Model file for the job. Use its own axes, mm. Face numbers are marked on the shaded views. A direction names the side the tool comes from. Round coordinates to 2 decimals unless told otherwise and drop trailing zeros. Order: outer loops, then holes, each group sorted by start corner. A loop starts at its lowest first (then second) coordinate and runs counter-clockwise, first axis right, second up. Notation, with made-up numbers: (79.5, 14) - (137.5, 14) arc R21 cw to (137.5, 50) - close; hole circle Ø7 at (18.5, 27). An arc over 180 degrees is marked (long way). Write item = value, one per line. Start each with the question number.
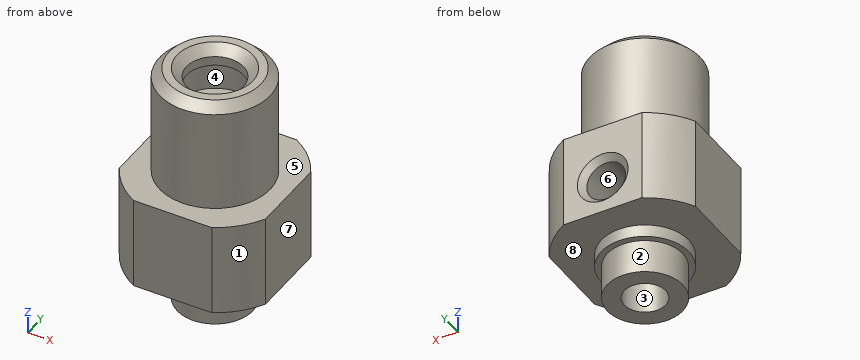
from build123d import *

# Parameters (mm, degrees)
CUT_EXTRUDE2_REACH              = 24
M5X0_8_TAPPED_HOLE1_D           = 4.2
M5X0_8_TAPPED_HOLE1_DEPTH       = 7
M5X0_8_TAPPED_HOLE1_CSINK_D     = 5.5
M5X0_8_TAPPED_HOLE1_CSINK_ANGLE = 90


with BuildPart() as part:
    # Sketch1 → Revolve1 (revolve)
    with BuildSketch(Plane(origin=(0, 0, 0), x_dir=(0, 0, -1), z_dir=(1, 0, 0))):
        Polygon((-12.5, 3.1), (-13.5, 4.1), (-13.5, 5), (-12.5, 6), (-1.5, 6), (-1.5, 9), (8.5, 9), (8.5, 4.75), (9.85, 4.75), (9.85, 4.1), (13.5, 4.1), (13.5, 2.25), (-8, 2.25), (-8, 4.15), (-11.5, 4.15), (-11.5, 3.1), align=None)
    revolve(axis=Axis((0, 0, 0), (0, 0, -1)))

    # Sketch2 → Cut-Extrude2 (cut, up to next)
    with BuildSketch(Plane(origin=(0, 0, -8.5), x_dir=(-1, 0, 0), z_dir=(0, 0, -1)), mode=Mode.PRIVATE) as cut_extrude2_sk1:
        with BuildLine():
            ThreePointArc((4.242180306, 7.9375), (0, 9), (-4.242180306, 7.9375))
            Line((-4.242180306, 7.9375), (4.242180306, 7.9375))
        make_face()
    cut_extrude2_tool1 = extrude(cut_extrude2_sk1.sketch, amount=-CUT_EXTRUDE2_REACH, mode=Mode.PRIVATE) & part.part
    add(cut_extrude2_tool1.solids().sort_by_distance((0, 8.364726, -8.5))[0], mode=Mode.SUBTRACT)
    # Sketch2 → Cut-Extrude2 (cut, up to next)
    with BuildSketch(Plane(origin=(0, 0, -8.5), x_dir=(-1, 0, 0), z_dir=(0, 0, -1)), mode=Mode.PRIVATE) as cut_extrude2_sk2:
        with BuildLine():
            Line((-7.9375, -4.242180306), (-7.9375, 4.242180306))
            ThreePointArc((-7.9375, 4.242180306), (-9, 0), (-7.9375, -4.242180306))
        make_face()
    cut_extrude2_tool2 = extrude(cut_extrude2_sk2.sketch, amount=-CUT_EXTRUDE2_REACH, mode=Mode.PRIVATE) & part.part
    add(cut_extrude2_tool2.solids().sort_by_distance((8.364726, 0, -8.5))[0], mode=Mode.SUBTRACT)
    # Sketch2 → Cut-Extrude2 (cut, up to next)
    with BuildSketch(Plane(origin=(0, 0, -8.5), x_dir=(-1, 0, 0), z_dir=(0, 0, -1)), mode=Mode.PRIVATE) as cut_extrude2_sk3:
        with BuildLine():
            Line((4.242180306, -7.9375), (-4.242180306, -7.9375))
            ThreePointArc((-4.242180306, -7.9375), (0, -9), (4.242180306, -7.9375))
        make_face()
    cut_extrude2_tool3 = extrude(cut_extrude2_sk3.sketch, amount=-CUT_EXTRUDE2_REACH, mode=Mode.PRIVATE) & part.part
    add(cut_extrude2_tool3.solids().sort_by_distance((0, -8.364726, -8.5))[0], mode=Mode.SUBTRACT)
    # Sketch2 → Cut-Extrude2 (cut, up to next)
    with BuildSketch(Plane(origin=(0, 0, -8.5), x_dir=(-1, 0, 0), z_dir=(0, 0, -1)), mode=Mode.PRIVATE) as cut_extrude2_sk4:
        with BuildLine():
            ThreePointArc((9, 0), (8.730335045, 2.186606961), (7.9375, 4.242180306))
            Line((7.9375, 4.242180306), (7.9375, -4.242180306))
            ThreePointArc((7.9375, -4.242180306), (8.730335045, -2.186606961), (9, 0))
        make_face()
    cut_extrude2_tool4 = extrude(cut_extrude2_sk4.sketch, amount=-CUT_EXTRUDE2_REACH, mode=Mode.PRIVATE) & part.part
    add(cut_extrude2_tool4.solids().sort_by_distance((-8.364726, 0, -8.5))[0], mode=Mode.SUBTRACT)

    # M5x0.8 Tapped Hole1
    with Locations(Plane(origin=(0, 7.9375, 0), x_dir=(1, 0, 0), z_dir=(0, 1, 0))):
        with Locations((0, 4.5)):
            CounterSinkHole(M5X0_8_TAPPED_HOLE1_D / 2, M5X0_8_TAPPED_HOLE1_CSINK_D / 2, depth=M5X0_8_TAPPED_HOLE1_DEPTH, counter_sink_angle=M5X0_8_TAPPED_HOLE1_CSINK_ANGLE)


solid = part.part
Item 1: Drop flat-ended pins along their axis: pin 1 (3 mm diameter, centred on y = -5.5, z = 9.5, fed in from -X); pin 2 (1 mm diameter, centred on x = -4.5, y = 1.5, fed in from -Z); pin 3 (2.5 mm diameter, centred on x = 1, y = 1, fed in from -Z); pin 4 (8 mm diameter, centred on x = 0, y = 0, fed in from +Z). Give the stop position or say it passes through.
Item 2: Probe L1, parallel to X at y = 0, z = 12.1; L2, parallel to X at y = 0, z = 10.8; L3, parallel to Z at x = -3, y = 6.5. List the from-to ranges inside material, lowest first.
Item 3: Saw through at D-D, the plane x = 0. Give the number of separate pieces and of enclosed holes in the cut face, then the cut area to 3 significant figures.
Item 4: Saw through at C-C, the plane z = -4.5. Give the cut face in (x, y), then the cut area to 3 significant figures.
Item 5: Mould opens along Y. For the marked faces 1, 2 and 3 say: +Y half, -Y half, draft (parallel to the pull), parting line (faces both ways), or undercut.
Item 6: Which spindle directions (+Z, -Z, +X, -X, +Y, -Y) get a long thin tool onto all of the face, cutting with end or side? Do the marked faces 4, 5, 6, 7 and 8. Say none if no direction does.
Item 7: Saw through at B-B, the plane z = -1.25. Give the cut face in (x, y).
Check sheet entries:
q1.pin_1 = -4.47
q1.pin_2 = -9.85
q1.pin_3 = -13.5
q1.pin_4 = 13.4
q2.L1 = -6 to -3.1, 3.1 to 6
q2.L2 = -6 to -4.15, 4.15 to 6
q2.L3 = -8.5 to 1.5
q3.separate_pieces = 3
q3.enclosed_holes = 0
q3.area = 181 mm2
q4.outline = (-7.94, -4.24) arc R9 ccw to (-4.24, -7.94) - (4.24, -7.94) arc R9 ccw to (7.94, -4.24) - (7.94, 4.24) arc R9 ccw to (4.24, 7.94) - (2.75, 7.94) - (2.1, 7.29) - (2.1, 0.94) - (2.05, 0.94) arc R2.25 cw (long way) to (-2.05, 0.94) - (-2.1, 0.94) - (-2.1, 7.29) - (-2.75, 7.94) - (-4.24, 7.94) arc R9 ccw to (-7.94, 4.24) - close
q4.area = 188 mm2
q5.face_1 = -Y half
q5.face_2 = parting line
q5.face_3 = undercut
q6.face_4 = none
q6.face_5 = +Z
q6.face_6 = +Y
q6.face_7 = +Z, -Z, +X, +Y, -Y
q6.face_8 = -Z
q7.outline = (-7.94, -4.24) arc R9 ccw to (-4.24, -7.94) - (4.24, -7.94) arc R9 ccw to (7.94, -4.24) - (7.94, 4.24) arc R9 ccw to (4.24, 7.94) - (-4.24, 7.94) arc R9 ccw to (-7.94, 4.24) - close; hole circle Ø4.5 at (0, 0)
